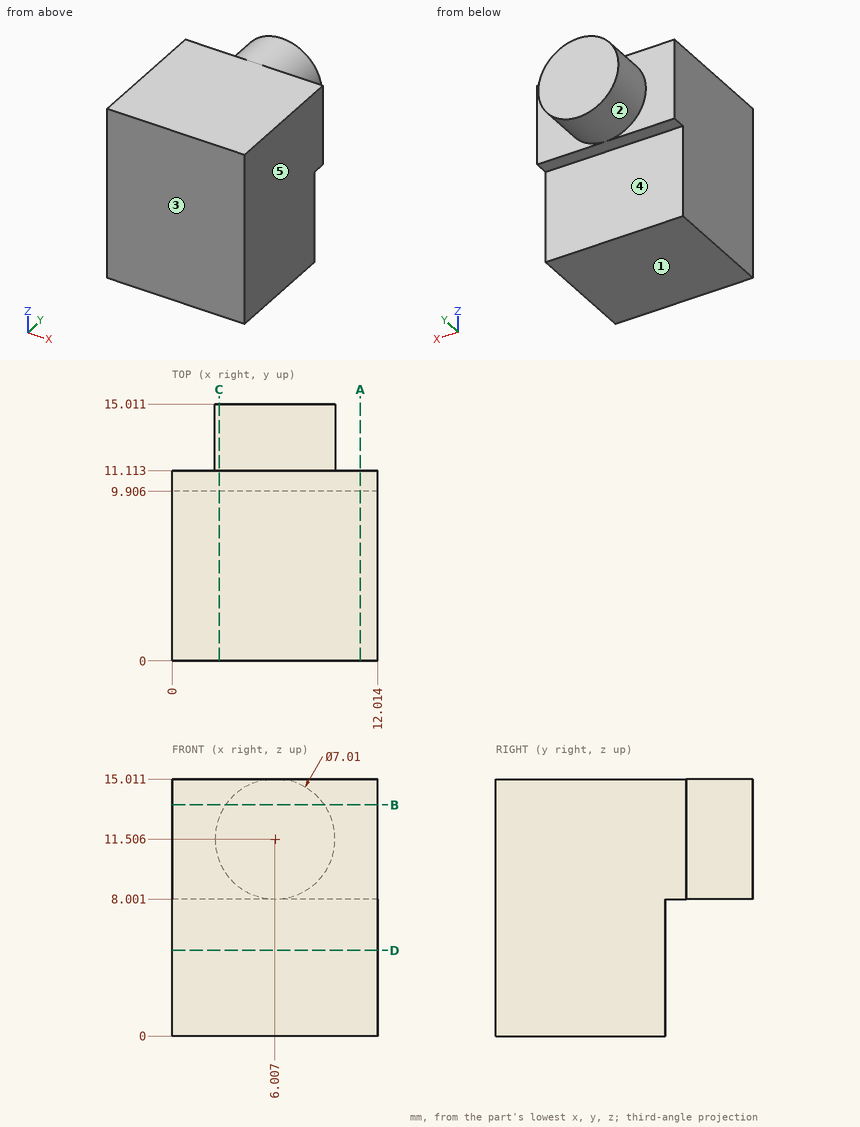
Check sheet for the drawn part. Datum: minimum x, y, z corner. Units: mm. A direction names the side the tool comes from. Coordinates: 2 decimals unless noted, no trailing zeros. Order: outer loops, then holes, each group sorted by start corner. A loop starts at its lowest first (then second) coordinate and runs counter-clockwise, first axis right, second up. Notation, with made-up numbers: (28, -40) - (41, -40) arc R8 cw to (41, -29) - close; hole circle Ø6 at (-12.5, 62.25). An arc over 180 degrees is marked (long way). Return JSON: item names as keys, results as strings.
(1) Section check D-D, the plane z = 5. Record the cut outline in (x, y) (1 decimal), and give its area (3 significant figures).
Filled sheet:
{"outline": "(0, 0) - (12, 0) - (12, 9.9) - (0, 9.9) - close", "area": "119 mm^2"}
(2) Section check A-A, the plane x = 11. Record the cut outline in (y, z) (1 decimal).
Filled sheet:
{"outline": "(0, 0) - (9.9, 0) - (9.9, 8) - (11.1, 8) - (11.1, 15) - (0, 15) - close"}
(3) Section check B-B, the plane z = 13.5. Record the cut outline in (x, y) (1 decimal).
Filled sheet:
{"outline": "(0, 0) - (12, 0) - (12, 11.1) - (8.9, 11.1) - (8.9, 15) - (3.1, 15) - (3.1, 11.1) - (0, 11.1) - close"}
(4) Access from +Z, -Z, +X, -X, +Y, -Y to the whole of each face (thin tool, end or side, straight path). Record for the marked faces 1 and 2.
Filled sheet:
{"face 1": "-Z, +X, -X, +Y, -Y", "face 2": "+Y"}
(5) Go/stop test with a flat-tipped pin: pin 1 (0.6 mm diameter, centred on x = 9, y = 10.5, fed in from -Z). Record where the tip stops, or that it passes through.
Filled sheet:
{"pin 1": "stops at z = 8"}
(6) Section check C-C, the plane x = 2.75. Record the cut outline in (y, z) (1 decimal).
Filled sheet:
{"outline": "(0, 0) - (9.9, 0) - (9.9, 8) - (11.1, 8) - (11.1, 10.2) - (15, 10.2) - (15, 12.8) - (11.1, 12.8) - (11.1, 15) - (0, 15) - close"}
(7) Thickness scan on line 1 along Y through (x, z) = (10.5, 12.5); line 2 along Y through (x, z) = (1.5, 5.75) (1 decimal); line 3 along Z through (x, y) = (7.75, 11). Record the ranges inside material, lowest first.
Filled sheet:
{"line 1": "y = 0 to 11.11", "line 2": "y = 0 to 9.9", "line 3": "z = 8 to 15.01"}
(8) Mould release check, pull along Y, two halves, no side actions. Record for the marked faces 3, 4 and 5: pulls with the +Y half, pulls with the -Y half, needs draft (parallel to the pull), parting line crosses it, or undercut.
Filled sheet:
{"face 3": "pulls with the -Y half", "face 4": "pulls with the +Y half", "face 5": "needs draft"}
